from build123d import *

# Parameters (mm, degrees)
F0_W     = 190
F0_H     = 39
F0_R     = 1.5
F1_DEPTH = 232
F2_W     = 2
F2_H     = 187
F2_H_2   = 2
F2_W_2   = 30
F3_DEPTH = 39
F4_W     = 160
F4_H     = 22
F5_DEPTH = 5
F6_R     = 10


with BuildPart() as f1:
    # F0 (on Top) → F1 (new body)
    with BuildSketch(Plane.XY):
        with Locations((95, 19.5)):
            Rectangle(F0_W, F0_H)
        with Locations((2, 20)):
            Circle(F0_R, mode=Mode.SUBTRACT)
        Polygon((188, 3), (2, 3), (2, 14.8786796564), (5, 17.8786796564), (5, 22.1213203436), (2, 25.1213203436), (2, 37), (188, 37), (188, 25.1213203436), (185, 22.1213203436), (185, 17.8786796564), (188, 14.8786796564), align=None, mode=Mode.SUBTRACT)
        with Locations((188, 20)):
            Circle(F0_R, mode=Mode.SUBTRACT)
    extrude(amount=F1_DEPTH)

    # F2 (on face) → F3 (join)
    with BuildSketch(Plane.XZ):
        with Locations((61, 138.5)):
            Rectangle(F2_W, F2_H)
        with Locations((61, 44)):
            Rectangle(F2_W, F2_H_2)
        with Locations((77, 44)):
            Rectangle(F2_W_2, F2_H_2)
    extrude(amount=-F3_DEPTH)

    # F4 (on face) → F5 (cut)
    with BuildSketch(Plane(origin=(0, 39, 0), x_dir=(-1, 0, 0), z_dir=(0, 1, 0))):
        Polygon((-95, 37), (-175, 22), (-15, 22), align=None)
        with Locations((-95, 11)):
            Rectangle(F4_W, F4_H)
    extrude(amount=-F5_DEPTH, mode=Mode.SUBTRACT)

    # F6
    f6_edges = [f1.edges().sort_by_distance(p)[0] for p in [
        (175, 38, 22),
        (15, 38, 22),
        (95, 38, 37),
    ]]
    fillet(f6_edges, radius=F6_R)


solid = f1.part
Input: part model. Units: mm. Frame: model coordinates. A direction names the side the tool comes from. Give positions to 0.01 mm unless a question says otherwise; leave off trailing zeros. Write each loop counter-clockwise with the first axis right and the second up, starting at its lowest first coordinate (ties: lowest second). Pieces come first, ordered by that corner, then holes. Notation, with made-up numbers: (33.25, 54) -> (59.25, 54) arc R28 ccw to (59.25, 76) -> close; hole circle Ø8 at (39.5, -38.5). An arc over 180 degrees is marked (long way). Use one line per item in the form item = value. Start each with the question number.
1) Section query A-A on y = 34. Return the cut outline in (x, z), then the cut area to 3 significant figures.
2) Ray query, probe 1 along X at (y, z) = (4.5, 140); probe 2 along Y at (x, z) = (132, 209); probe 3 along X at (y, z) = (17, 49). Return the intervals inside material, ascending. Write a range as from..to.
3) Set-up query: faces 1 (the flat face through (60, 20, 139)), 2 (the flat face through (76, 20, 43)), 3 (the flat face through (77, 20, 45)), 4 (the cylindrical face through (172.76, 37.99, 20.01)), 5 (the flat face through (94, 39, 114)). Return all of +Z, -Z, +X, -X, +Y, -Y with unobstructed straight access to the full face (end or side cutting, diameter ignored); none if empty.
4) Section query B-B on z = 175.5. Return the cut outline in (x, y), then the cut area to 3 significant figures.
5) Pin query (flat end, axial travel): pin 1 (4 mm diameter, centred on x = 84, y = 29.5, fed in from +Z). Return the tip coordinate at first contact, or that it passes through.
6) Section query C-C on x = 18. Return the cut outline in (y, z), then the cut area to 3 significant figures.
7) Draft query along X for faces 6 (the cylindrical face through (17.24, 37.99, 20.01)), 7 (the flat face through (57.67, 38.01, 30)), 8 (the flat face through (95, 2, 232)), 9 (the flat face through (190, 19, 114)). Return one class per face: pulls with the +X half, pulls with the -X half, needs draft (parallel to the pull), parting line crosses it, or undercut.
Outcome:
q1.outline = (0, 0) -> (2, 0) -> (2, 232) -> (0, 232) -> close; (60, 43) -> (92, 43) -> (92, 45) -> (62, 45) -> (62, 232) -> (60, 232) -> close; (188, 0) -> (190, 0) -> (190, 232) -> (188, 232) -> close
q1.area = 1,370 mm^2
q2.probe_1 = 0..2, 60..62, 188..190
q2.probe_2 = 0..3, 37..39
q2.probe_3 = 0..4.12, 60..62, 185.88..190
q3.face_1 = +Z, -Z
q3.face_2 = -Z
q3.face_3 = +Z
q3.face_4 = -Z, +Y
q3.face_5 = +Z, -Z, +X, -X, +Y
q4.outline = (0, 0) -> (190, 0) -> (190, 39) -> (0, 39) -> close; hole circle Ø3 at (2, 20); hole (2, 3) -> (60, 3) -> (60, 37) -> (2, 37) -> (2, 25.12) -> (5, 22.12) -> (5, 17.88) -> (2, 14.88) -> close; hole (62, 3) -> (188, 3) -> (188, 14.88) -> (185, 17.88) -> (185, 22.12) -> (188, 25.12) -> (188, 37) -> (62, 37) -> close; hole circle Ø3 at (188, 20)
q4.area = 1,180 mm^2
q5.pin_1 = 45
q6.outline = (0, 0) -> (3, 0) -> (3, 232) -> (0, 232) -> close; (37, 20.84) -> (39, 20.84) -> (39, 232) -> (37, 232) -> close
q6.area = 1,120 mm^2
q7.face_6 = undercut
q7.face_7 = undercut
q7.face_8 = needs draft
q7.face_9 = pulls with the +X half
